Autodesk Inventor part; units mm, degrees
ref_plane "YZ Plane" through (0, 0, 0) normal (1, 0, 0) x (0, 1, 0)
ref_plane "XZ Plane" through (0, 0, 0) normal (0, 1, 0) x (-1, 0, 0)
ref_plane "XY Plane" through (0, 0, 0) normal (0, 0, 1) x (1, 0, 0)
sketch "Sketch3" plane through (0, 0, 0) normal (1, 0, 0) x (0, 1, 0)
  circle A0 centre (0, 0) radius 1.6
  arc A1 (1.725, -2.4545) -> (-1.6531, -2.5034) centre (0, 0) ccw
  line L0 (-0.7552, -4.1724) -> (-0.7552, -12)
  line L1 (-0.7552, -12) -> (0.875, -12)
  line L2 (0.875, -12) -> (0.875, -4.0908)
  arc A2 (1.725, -2.4545) -> (0.875, -4.0908) centre (2.875, -4.0908) ccw
  arc A3 (-0.7552, -4.1724) -> (-1.6531, -2.5034) centre (-2.7552, -4.1724) ccw
  dimension "d4" = 3.2
  dimension "d5" = 6
  dimension "d7" = 2
  dimension "d33" = 12
extrude "Extrusion2" add sketch "Sketch3" along normal blind 30
sketch "Sketch5" plane through (0, 0.875, -4.0908) normal (0, 1, 0) x (1, 0, 0)
  line L0 (0, 7.9092) -> (30, 7.9092)
  line L1 (6, 7.9092) -> (24, 7.9092)
  line L2 (24, 7.9092) -> (24, 1.9092)
  line L3 (24, 1.9092) -> (6, 1.9092)
  line L4 (6, 1.9092) -> (6, 7.9092)
  line L5 (0, 7.9092) -> (0, 0)
  point P0 (0, -4.0908)
  dimension "d18" = 6
  dimension "d19" = 30
  dimension "d20" = 6
  dimension "d21" = 18
extrude "Extrusion3" cut sketch "Sketch5" along normal blind 0.5 and the other way blind 2
chamfer "Chamfer3" distance 4 angle 45 2 edges at (6, 0.0599, -12) (24, 0.0599, -12)
fillet "Fillet1" radius 2 4 edges at (30, 0.0599, -12) (0, 0.0599, -12) (24, 0.0599, -6) (6, 0.0599, -6)
chamfer "Chamfer2" distance 0.25 angle 45 28 edges at (6, 0.875, -7.9998) (6.5856, 0.875, -6.5856) (23.4144, 0.875, -6.5856) (24, 0.875, -7.9998) (29.4144, 0.875, -11.4144) (30, 0.875, -7.0456) (30, 1.1002, -3.1688) (30, -0.0435, 2.9997) (30, -0.9939, -3.2248) (30, -0.7552, -7.0865) (29.4144, -0.7552, -11.4144) (23.4144, -0.7552, -6.5856) (24, -0.7552, -7.9997) (6, -0.7552, -7.9998) (6.5856, -0.7552, -6.5856) (0.5856, -0.7552, -11.4144) (0, -0.7552, -7.0865) (0, -0.9939, -3.2248) (0, -0.0435, 2.9997) (0, 1.1002, -3.1688) (0, 0.875, -7.0456) (0.5856, 0.875, -11.4144) (30, -1.6, 0) (0, -1.6, 0) (26, 0.875, -10) (26, -0.7552, -10) (4, 0.875, -10) (4, -0.7552, -10)
equation "\"d20\" = -0.5 * d21 + 0.5 * d19"
properties part number "CoinLockUpperRow2"
Here's how the part is built. I have some questions about the finished solid (model axes, mm). A direction names the side the tool comes from. Give positions to 0.01 mm unless a question says otherwise; leave off trailing zeros. Order: outer loops, then holes, each group sorted by start corner. A loop starts at its lowest first (then second) coordinate and runs counter-clockwise, first axis right, second up. Notation, with made-up numbers: M 5,41 L 27,41 A20 cw 27,61 Z; hole C -21.5,37 d5. An arc over 180 degrees is marked long. Answer as a JSON object with one key per item and string values. Group by question number.
1) I'm going to push flat-ended pins straight in: pin 1 Ø1 at (x, y) = (9, 0.5) entering from -Z; pin 2 Ø1.5 at (x, z) = (26.5, -4) entering from -Y; pin 3 Ø2.5 at (y, z) = (0, 0) entering from +X; pin 4 Ø2.5 at (x, z) = (18.5, -6.5) entering from -Y. Where does each tip first touch, or does it pass through?
2) We'd pull the mould along X, two halves only. Please class faces 6 (the flat face through (26, 0, -10)), 7 (the cylindrical face through (14.79, -1.27, 0.97)), 8 (the conical face through (29.31, 0.75, -11.34)): pulls with the +X half, pulls with the -X half, needs draft (parallel to the pull), parting line crosses it, or undercut.
3) On a 3-axis mill with a long thin cutter (end or side, diameter ignored), from which of +Z, -Z, +X, -X, +Y, -Y can I reach the whole of each face in a straight line? I mean faces 1 (the flat face through (15, -0.755, -5)), 2 (the flat face through (3.88, 0.75, -9.94)), 3 (the flat face through (3.88, -0.63, -9.94)), 4 (the cylindrical face through (23.43, 0.05, -6.6)), 5 (the cylindrical face through (15, 0, 3)). Say none if no direction works.
4) Suppose I cut it at B-B, the plane x = 26. Write out the boundary of the cut face in (y, z) (1 decimal).
5) Please list where these lines run through material, in increasing order: L1, parallel to Z at x = 9.25, y = 0; L2, parallel to Z at x = 25, y = 0.5; L3, parallel to X at y = 0.25, z = -10.5. Write a range as [from, to].
Results found:
{
 "1": {"pin 1": "z = -6", "pin 2": "y = -0.98", "pin 3": "through", "pin 4": "y = -0.76"},
 "2": {"face 6": "undercut", "face 7": "needs draft", "face 8": "pulls with the +X half"},
 "3": {"face 1": "-Z, +X, -X, -Y", "face 2": "-Z, +Y", "face 3": "-Z, -Y", "face 4": "-Z, +Y, -Y", "face 5": "+X, -X"},
 "4": {"outline": "M -1.7,-2.5 A2 cw -0.8,-4.2 L -0.8,-9.6 L -0.5,-10 L 0.6,-10 L 0.9,-9.6 L 0.9,-4.1 A2 cw 1.7,-2.5 A3 ccw long Z; hole C 0,0 d3.2"},
 "5": {"L1": "[-6, -1.6], [1.6, 3]", "L2": "[-9, -1.52], [1.52, 2.96]", "L3": "[0.06, 3.5], [26.5, 29.94]"}
}
